The listing builds one solid part. Answer for the finished solid, in the listing's coordinates (mm). A direction names the side the tool comes from. Round coordinates to 2 decimals unless told otherwise and drop trailing zeros. Order: outer loops, then holes, each group sorted by start corner. A loop starts at its lowest first (then second) coordinate and runs counter-clockwise, first axis right, second up. Notation, with made-up numbers: (-34.75, -26) - (10.25, -26) arc R33 ccw to (10.25, 9) - close; hole circle Ø9 at (-7, -32.75). An arc over 180 degrees is marked (long way). Use CSV: the item, a comma, the result in double quotes. Start each with the question number.
Item 1: Find section B-B, the plane z = 2. Give the vertices of the cut face in (x, y), plus the area to 3 significant figures.
Item 2: Find section C-C, the plane y = 0. Give the vertices of the cut face in (x, z).
Item 3: Straight lines are drawn through the part: line 1 along Y through (x, z) = (-7.5, 1.85); line 2 along Z through (x, y) = (-8.25, 2.3); line 3 along X through (y, z) = (-1.4, 29). For each, find the intervals that lie inside material, in ascending order. Write a range as [from, to].
Item 4: Determine the mould class of faces 1 (the flat face through (2, 0, 20)), 2 (the flat face through (0, 0, 0)), 3 (the flat face through (-9, 1, 33.5)), 4 (the cylindrical face through (-2.45, 0.04, 33.07)) for opening direction Z: +Z half, -Z half, draft (parallel to the pull), parting line (faces both ways), or undercut.
Item 5: For faces 5 (the flat face through (8, 2, 3)), 6 (the flat face through (-2, 0, 18)), 7 (the flat face through (-12, 0, 35)), determine the directions among +Z, -Z, +X, -X, +Y, -Y from which every point of the face is accessible in a straight line to the end or side of a thin tool.
Item 6: Flat-ended cylindrical pins translate along their axes: P1, Ø1.5, axis at y = 1, z = 14, coming from the -X side; P2, Ø3, axis at x = -7.5, y = 0, coming from the -Z side; P3, Ø2, axis at y = 0, z = 6.5, coming from the +X side; P4, Ø2, axis at x = 7.5, y = 0, coming from the +Z side. Find the tip coordinate at first contact, or state that the pin passes through.
Item 7: Find section D-D, the plane x = -7.5. Give the vertices of the cut face in (y, z), plus the area to 3 significant figures.
Item 8: Find section A-A, the plane x = 7.5. Give the vertices of the cut face in (y, z), plus the area to 3 significant figures.
```python
from build123d import *

# Parameters (mm, degrees)
SKETCH1_W           = 25
SKETCH1_H           = 5
SKETCH1_R           = 1.75
BOSS_EXTRUDE1_DEPTH = 3
SKETCH2_W           = 4
SKETCH2_H           = 5
BOSS_EXTRUDE2_DEPTH = 33.5
SKETCH3_W           = 3
SKETCH3_H           = 5
BOSS_EXTRUDE3_DEPTH = 10
SKETCH4_R           = 1.75
CUT_EXTRUDE1_DEPTH  = 10
FILLET1_R           = 1.5


with BuildPart() as part:
    # Sketch1 → Boss-Extrude1 (new body)
    with BuildSketch(Plane.XY):
        Rectangle(SKETCH1_W, SKETCH1_H)
        with Locations((-7.5, 0)):
            Circle(SKETCH1_R, mode=Mode.SUBTRACT)
        with Locations(Location((7.5, 0, 0), (0, 0, 180))):
            Circle(SKETCH1_R, mode=Mode.SUBTRACT)
    extrude(amount=BOSS_EXTRUDE1_DEPTH)

    # Sketch2 → Boss-Extrude2 (add)
    with BuildSketch(Plane.XY.offset(3)):
        Rectangle(SKETCH2_W, SKETCH2_H)
    extrude(amount=BOSS_EXTRUDE2_DEPTH)

    # Sketch3 → Boss-Extrude3 (add)
    with BuildSketch(Plane.ZY.offset(2)):
        with Locations((35, 0)):
            Rectangle(SKETCH3_W, SKETCH3_H)
    extrude(amount=BOSS_EXTRUDE3_DEPTH)

    # Sketch4 → Cut-Extrude1 (cut)
    with BuildSketch(Plane(origin=(0, 0, 33.5), x_dir=(-1, 0, 0), z_dir=(0, 0, -1))):
        with Locations((7, 0)):
            Circle(SKETCH4_R)
    extrude(amount=-CUT_EXTRUDE1_DEPTH, mode=Mode.SUBTRACT)

    # Fillet1
    fillet1_edges = [part.edges().sort_by_distance(p)[0] for p in [
        (-2, 0, 3),
        (2, 0, 3),
        (2, 0, 36.5),
        (-2, 0, 33.5),
    ]]
    fillet(fillet1_edges, radius=FILLET1_R)


solid = part.part
```
Worked out:
1,outline,"(-12.5, -2.5) - (12.5, -2.5) - (12.5, 2.5) - (-12.5, 2.5) - close; hole circle Ø3.5 at (-7.5, 0); hole circle Ø3.5 at (7.5, 0)"
1,area,"106 mm²"
2,outline,"(-12.5, 0) - (-9.25, 0) - (-9.25, 3) - (-12.5, 3) - close; (-12, 33.5) - (-8.75, 33.5) - (-8.75, 36.5) - (-12, 36.5) - close; (-5.75, 0) - (5.75, 0) - (5.75, 3) - (3.5, 3) arc R1.5 cw to (2, 4.5) - (2, 35) arc R1.5 ccw to (0.5, 36.5) - (-5.25, 36.5) - (-5.25, 33.5) - (-3.5, 33.5) arc R1.5 cw to (-2, 32) - (-2, 4.5) arc R1.5 cw to (-3.5, 3) - (-5.75, 3) - close; (9.25, 0) - (12.5, 0) - (12.5, 3) - (9.25, 3) - close"
3,line 1,"y = [-2.5, -1.75], [1.75, 2.5]"
3,line 2,"z = [0, 3], [33.5, 36.5]"
3,line 3,"x = [-2, 2]"
4,face 1,"draft"
4,face 2,"-Z half"
4,face 3,"undercut"
4,face 4,"undercut"
5,face 5,"+Z, +X, +Y, -Y"
5,face 6,"-X, +Y, -Y"
5,face 7,"+Z, -X, +Y, -Y"
6,P1,"stops at x = -2"
6,P2,"stops at z = 33.5"
6,P3,"stops at x = 2"
6,P4,"passes through"
7,outline,"(-2.5, 0) - (-1.75, 0) - (-1.75, 3) - (-2.5, 3) - close; (-2.5, 33.5) - (-1.68, 33.5) - (-1.68, 36.5) - (-2.5, 36.5) - close; (1.68, 33.5) - (2.5, 33.5) - (2.5, 36.5) - (1.68, 36.5) - close; (1.75, 0) - (2.5, 0) - (2.5, 3) - (1.75, 3) - close"
7,area,"9.44 mm²"
8,outline,"(-2.5, 0) - (-1.75, 0) - (-1.75, 3) - (-2.5, 3) - close; (1.75, 0) - (2.5, 0) - (2.5, 3) - (1.75, 3) - close"
8,area,"4.50 mm²"
